Geometry check sheet. Reference: drawing and pictorial views, mm from the part's lowest x, y, z. Give positions to 0.01 mm unless a question says otherwise; leave off trailing zeros. Loops run counter-clockwise (first coordinate to the right, second up) from the corner with the lowest first, then second, coordinate; pieces in that order, holes last. Notation, with made-up numbers: (-9, 5) - (35, 5) arc R23 ccw to (35, 22) - close; hole circle Ø7 at (-8, 19.5). An arc over 180 degrees is marked (long way). Answer in a Markdown table with one row per item. Add a question column.
(1) Thickness scan on L1, parallel to X at y = 51, z = 100; L2, parallel to Y at x = 100, z = 112; L3, parallel to Y at x = 122, z = 108. Record the ranges inside material, lowest first.
(2) Sectioned sample at D-D on x = 187.5. Enter the section's corners in (y, z).
(3) Go/stop test with flat-tipped pins: P1, Ø2, axis at x = 166.5, z = 102.5, coming from the -Y side; P2, Ø2.5, axis at x = 100, y = 73.38, coming from the +Z side; P3, Ø8, axis at x = 84.5, y = 29, coming from the +Z side; P4, Ø1.5, axis at x = 116, z = 83.5, coming from the +Y side. Record where each tip stops, or that it passes through.
(4) Sectioned sample at C-C on y = 16. Enter the section's corners in (x, z).
(5) Sectioned sample at B-B on y = 63.5. Enter the section's corners in (x, z).
(6) Draft check along X on the marked faces 1, 2 and 3. Enter one of: released by +X, released by -X, zero draft, split by the parting line, or undercut.
(7) Sectioned sample at A-A on z = 100. Enter the section's corners in (x, y), then the cut area to 3 significant figures.
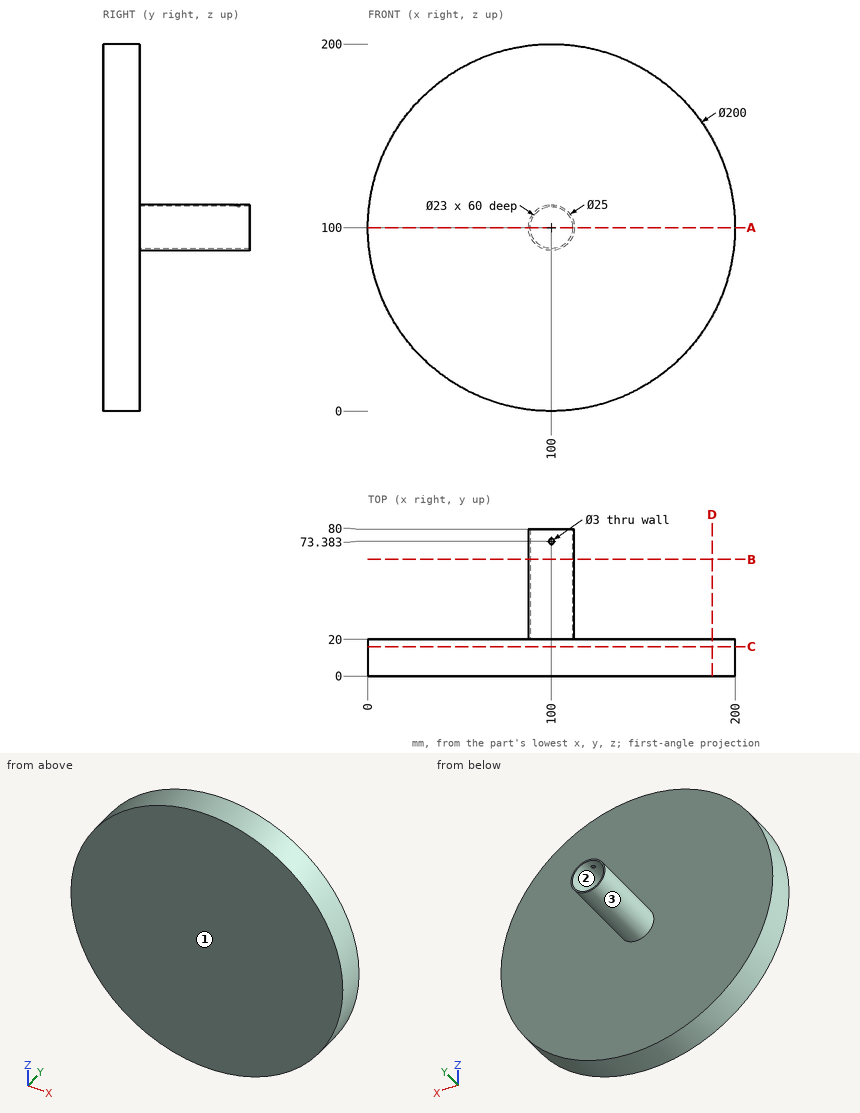
Reply:
| question | item | result |
|---|---|---|
| 1 | L1 | 87.5 to 88.5, 111.5 to 112.5 |
| 1 | L2 | 0 to 71.88, 74.88 to 80 |
| 1 | L3 | 0 to 20 |
| 2 | outline | (0, 51.59) - (20, 51.59) - (20, 148.41) - (0, 148.41) - close |
| 3 | P1 | y = 0 |
| 3 | P2 | z = 88.57 |
| 3 | P3 | z = 104.9 |
| 3 | P4 | y = 20 |
| 4 | outline | circle Ø200 at (100, 100) |
| 5 | outline | circle Ø25 at (100, 100); hole circle Ø23 at (100, 100) |
| 6 | face 1 | zero draft |
| 6 | face 2 | undercut |
| 6 | face 3 | split by the parting line |
| 7 | outline | (0, 0) - (200, 0) - (200, 20) - (112.5, 20) - (112.5, 80) - (111.5, 80) - (111.5, 20) - (88.5, 20) - (88.5, 80) - (87.5, 80) - (87.5, 20) - (0, 20) - close |
| 7 | area | 4,120 mm^2 |
